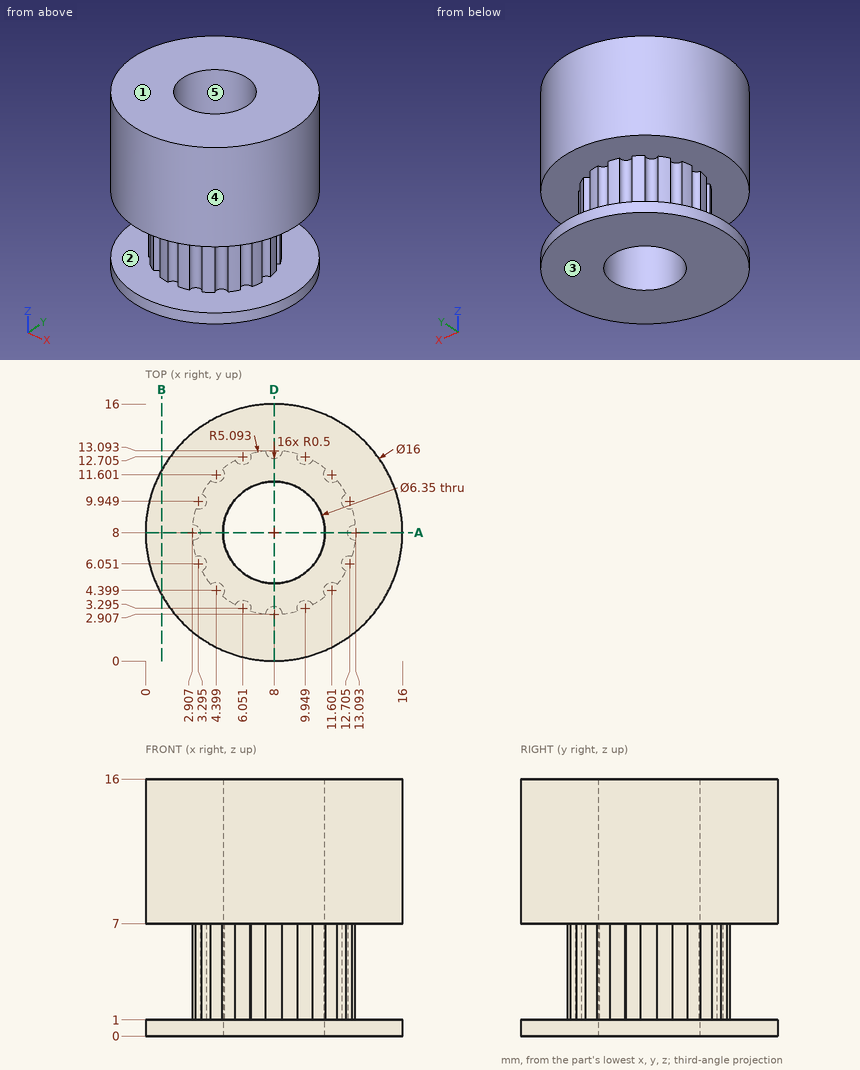
Design review of the part shown in the three views and the two pictorial views. Dimensions are in mm from the part's minimum x, y and z. A direction names the side the tool comes from. Round coordinates to 2 decimals unless told otherwise and drop trailing zeros. Loops run counter-clockwise (first coordinate to the right, second up) from the corner with the lowest first, then second, coordinate; pieces in that order, holes last.
(1) Wall thickness on line 1 along Z through (x, y) = (4, 14.5); line 2 along Y through (x, z) = (8, 11) (1 decimal); line 3 along Y through (x, z) = (8, 5.5) (1 decimal): over which ranges is each line inside the solid? List them lowest first.
Returned:
line 1: z = 0 to 1, 7 to 16
line 2: y = 0 to 4.8, 11.2 to 16
line 3: y = 3.4 to 4.8, 11.2 to 12.6
(2) Tool access review of the marked faces 1 and 2: name each direction out of +Z, -Z, +X, -X, +Y, -Y from which nothing blocks a thin tool from reaching the whole face with its end or side.
Returned:
face 1: +Z, +X, -X, +Y, -Y
face 2: none
(3) Clearance check with flat-ended pins moving along their axes: P1, Ø6, axis at x = 6.5, z = 10, coming from the +Y side; P2, Ø2, axis at y = 11.5, z = 2.5, coming from the -X side. State where each tip first meets the part, or that it passes through.
Returned:
P1: stops at y = 16
P2: stops at x = 3.56
(4) We need section A-A (y = 8). Give the boundary of the cut face in (x, z) (1 decimal).
Returned:
outline: (0, 0) - (4.8, 0) - (4.8, 16) - (0, 16) - (0, 7) - (3.4, 7) - (3.4, 1) - (0, 1) - close; (11.2, 0) - (16, 0) - (16, 1) - (12.6, 1) - (12.6, 7) - (16, 7) - (16, 16) - (11.2, 16) - close
(5) Mouldability with a two-part tool opening along Y and no side actions: class the marked faces 3, 4 and 5 as released by +Y, released by -Y, zero draft, split by the parting line, or undercut.
Returned:
face 3: zero draft
face 4: split by the parting line
face 5: undercut
(6) We need section B-B (x = 1). Give the boundary of the cut face in (y, z).
Returned:
outline: (4.13, 0) - (11.87, 0) - (11.87, 1) - (4.13, 1) - close; (4.13, 7) - (11.87, 7) - (11.87, 16) - (4.13, 16) - close
